Part model, mm, in its own coordinate system. Face numbers are marked on the shaded views. Coordinates: 2 decimals unless noted, no trailing zeros. Order: outer loops, then holes, each group sorted by start corner. A loop starts at its lowest first (then second) coordinate and runs counter-clockwise, first axis right, second up.
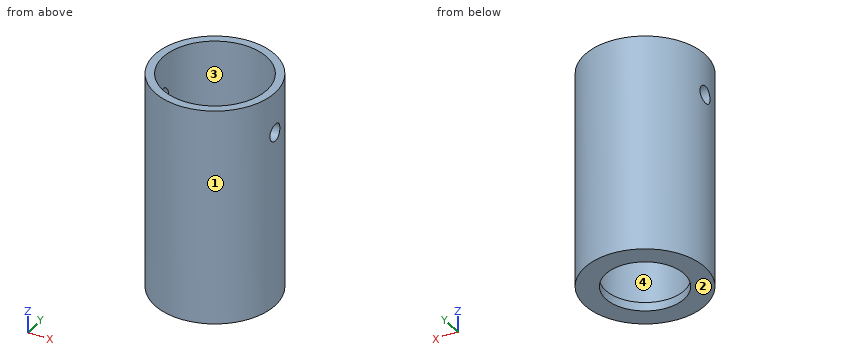
```python
from build123d import *

# Parameters (mm, degrees)
F0_R     = 14
F0_R_2   = 12.1
F1_DEPTH = 27.5
F2_R     = 14
F2_R_2   = 4.5
F3_DEPTH = 5
F4_R     = 14
F4_R_2   = 10
F5_DEPTH = 16
F6_R     = 14
F6_R_2   = 9.15
F7_DEPTH = 2
F8_R     = 2
F9_DEPTH = 20


with BuildPart() as f1:
    # F0 (on Top) → F1 (new body)
    with BuildSketch(Plane.XY):
        Circle(F0_R)
        Circle(F0_R_2, mode=Mode.SUBTRACT)
    extrude(amount=F1_DEPTH)

    # F2 (on Top) → F3 (join)
    with BuildSketch(Plane.XY):
        Circle(F2_R)
        Circle(F2_R_2, mode=Mode.SUBTRACT)
    extrude(amount=-F3_DEPTH)

    # F4 (on face) → F5 (join)
    with BuildSketch(Plane(origin=(0, 0, -5), x_dir=(1, 0, 0), z_dir=(0, 0, -1))):
        Circle(F4_R)
        Circle(F4_R_2, mode=Mode.SUBTRACT)
    extrude(amount=F5_DEPTH)

    # F6 (on face) → F7 (join)
    with BuildSketch(Plane(origin=(0, 0, -21), x_dir=(1, 0, 0), z_dir=(0, 0, -1))):
        Circle(F6_R)
        Circle(F6_R_2, mode=Mode.SUBTRACT)
    extrude(amount=F7_DEPTH)

    # F8 (on Right) → F9 (cut, symmetric)
    with BuildSketch(Plane.YZ):
        with Locations((0, 18)):
            Circle(F8_R)
    extrude(amount=F9_DEPTH, both=True, mode=Mode.SUBTRACT)


solid = f1.part
```
(1) Pull direction Y, two halves, no side cores. Call the marked faces 1, 2, 3 and 4: +Y half, -Y half, draft (parallel to the pull), parting line (faces both ways), or undercut.
(2) Slice it at A-A, the plane x = 0. Give the cut face in (y, z).
(3) Probe line 1 (X direction, y = 0, z = -22.45); line 2 (Z direction, x = -1.25, y = 9.25); line 3 (Y direction, x = 0, z = -1.3). List the from-to ranges inside material, lowest first.
(4) Slice it at D-D, the plane z = -17. Give the cut face in (x, y).
(5) Slice it at B-B, the plane y = 0. Give the cut face in (x, z).
(6) Drop flat-ended pins along their axis: pin 1 (1.5 mm diameter, centred on y = -5.5, z = -8, fed in from -X); pin 2 (1 mm diameter, centred on x = 2.5, z = 15.5, fed in from -Y); pin 3 (2 mm diameter, centred on y = -9.5, z = -13.5, fed in from +X); pin 4 (3.5 mm diameter, centred on y = 0, z = 18, fed in from +X). Give the stop position or say it passes through.
Here are the results:
1. face 1: parting line
1. face 2: draft
1. face 3: undercut
1. face 4: undercut
2. outline: (-14, -23) - (-9.15, -23) - (-9.15, -21) - (-10, -21) - (-10, -5) - (-4.5, -5) - (-4.5, 0) - (-12.1, 0) - (-12.1, 27.5) - (-14, 27.5) - close; (4.5, -5) - (10, -5) - (10, -21) - (9.15, -21) - (9.15, -23) - (14, -23) - (14, 27.5) - (12.1, 27.5) - (12.1, 0) - (4.5, 0) - close
3. line 1: x = -14 to -9.15, 9.15 to 14
3. line 2: z = -23 to -21, -5 to 0
3. line 3: y = -14 to -4.5, 4.5 to 14
4. outline: circle Ø28 at (0, 0); hole circle Ø20 at (0, 0)
5. outline: (-14, -23) - (-9.15, -23) - (-9.15, -21) - (-10, -21) - (-10, -5) - (-4.5, -5) - (-4.5, 0) - (-12.1, 0) - (-12.1, 16) - (-14, 16) - close; (-14, 20) - (-12.1, 20) - (-12.1, 27.5) - (-14, 27.5) - close; (4.5, -5) - (10, -5) - (10, -21) - (9.15, -21) - (9.15, -23) - (14, -23) - (14, 16) - (12.1, 16) - (12.1, 0) - (4.5, 0) - close; (12.1, 20) - (14, 20) - (14, 27.5) - (12.1, 27.5) - close
6. pin 1: stops at x = -13.17
6. pin 2: stops at y = -13.86
6. pin 3: stops at x = 11.12
6. pin 4: passes through
